Check sheet for the drawn part. Datum: minimum x, y, z corner. Units: mm. A direction names the side the tool comes from. Coordinates: 2 decimals unless noted, no trailing zeros. Write each loop counter-clockwise with the first axis right and the second up, starting at its lowest first coordinate (ties: lowest second). Pieces come first, ordered by that corner, then holes. Notation, with made-up numbers: M 67.25,-28.75 L 86.25,-28.75 A14 ccw 86.25,-20.75 Z; hole C 67,9 d6. An arc over 180 degrees is marked long. Answer in a Markdown table with one row per item.
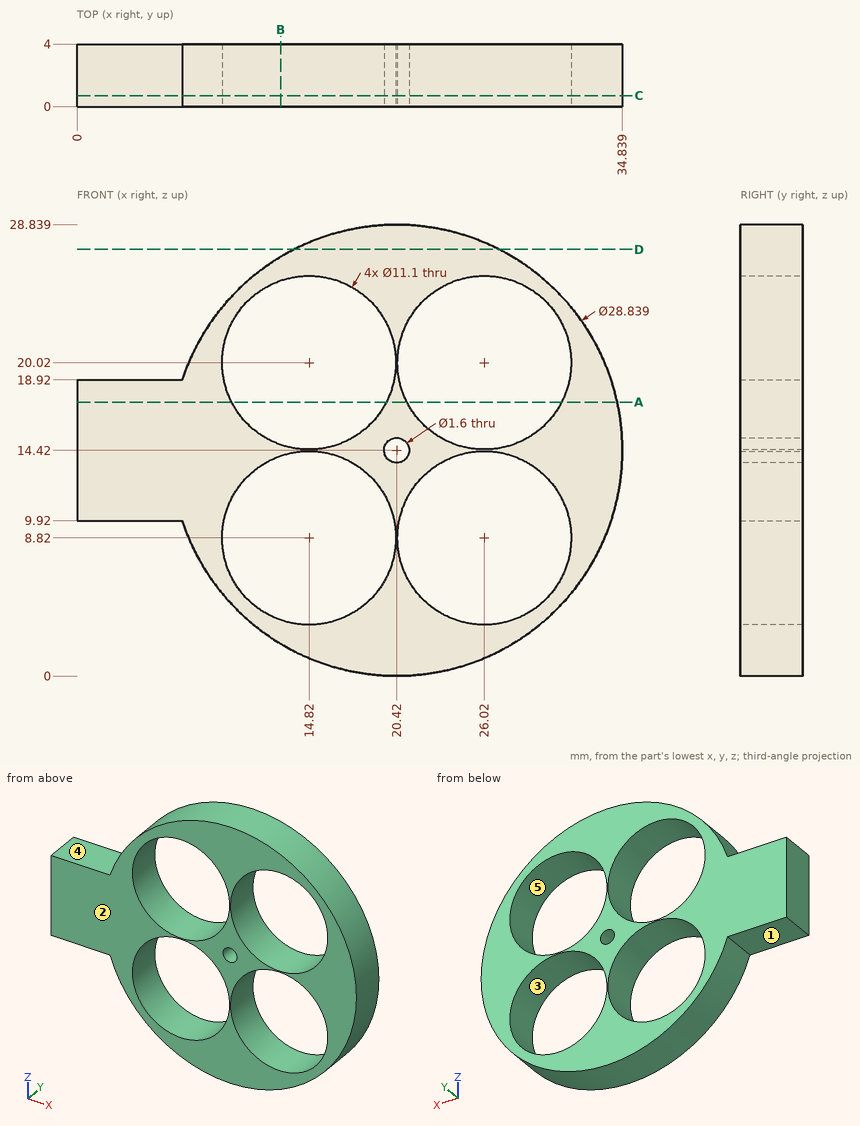
1) Sectioned sample at C-C (y = 0.7). Record the cut outline in (x, z).
Response values:
| item | result |
|---|---|
| outline | M 0,9.92 L 6.72,9.92 A14.42 ccw long 6.72,18.92 L 0,18.92 Z; hole C 14.82,8.82 d11.1; hole C 14.82,20.02 d11.1; hole C 20.42,14.42 d1.6; hole C 26.02,8.82 d11.1; hole C 26.02,20.02 d11.1 |
2) Release check for a two-part mould opening along Z. For the marked faces 1, 2 and 3 record: +Z half, -Z half, draft (parallel to the pull), parting line (faces both ways), or undercut.
Response values:
| item | result |
|---|---|
| face 1 | -Z half |
| face 2 | draft |
| face 3 | undercut |
3) Tool access check on the marked faces 4 and 5. Record the directions out of +Z, -Z, +X, -X, +Y, -Y that give a thin tool (end or side, any length) a straight path to the whole face; none if there is none.
Response values:
| item | result |
|---|---|
| face 4 | +Z, -X, +Y, -Y |
| face 5 | +Y, -Y |
4) Sectioned sample at A-A (z = 17.5). Record the cut outline in (x, y) (1 decimal).
Response values:
| item | result |
|---|---|
| outline | M 0,0 L 9.9,0 L 9.9,4 L 0,4 Z; M 19.8,0 L 21.1,0 L 21.1,4 L 19.8,4 Z; M 31,0 L 34.5,0 L 34.5,4 L 31,4 Z |
5) Sectioned sample at D-D (z = 27.25). Record the cut outline in (x, y).
Response values:
| item | result |
|---|---|
| outline | M 13.84,0 L 27,0 L 27,4 L 13.84,4 Z |
6) Thickness scan on L1, parallel to Z at x = 31, y = 2.2 (1 decimal); L2, parallel to Z at x = 29.5, y = 2.45 (1 decimal); L3, parallel to X at y = 2.8, z = 22 (1 decimal). Record the ranges inside material, lowest first. Write a range as [from, to].
Response values:
| item | result |
|---|---|
| L1 | z = [4.6, 6.4], [11.3, 17.6], [22.5, 24.2] |
| L2 | z = [3.2, 4.5], [13.1, 15.7], [24.3, 25.6] |
| L3 | x = [8.2, 9.6], [20, 20.8], [31.2, 32.7] |
7) Depth check by flat-ended pin: pin 1 (1.5 mm diameter, centred on y = 2, z = 9.5, fed in from +X); pin 2 (1 mm diameter, centred on y = 0.5, z = 24.5, fed in from -X). Enter the tip coordinate at first touch or a pass-through.
Response values:
| item | result |
|---|---|
| pin 1 | stops at x = 34.22 |
| pin 2 | stops at x = 9.64 |
8) Sectioned sample at B-B (x = 13). Record the cut outline in (y, z) (1 decimal), then the cut area to 3 significant figures.
Response values:
| item | result |
|---|---|
| outline | M 0,2.1 L 4,2.1 L 4,3.6 L 0,3.6 Z; M 0,14.1 L 4,14.1 L 4,14.8 L 0,14.8 Z; M 0,25.3 L 4,25.3 L 4,26.8 L 0,26.8 Z |
| area | 15.0 mm² |
